from build123d import *

# Parameters (mm, degrees)
BOSS_EXTRUDE1_DEPTH = 10
SKETCH2_R           = 2
CUT_EXTRUDE1_DEPTH  = 30
SKETCH4_W           = 18.757466853
SKETCH4_H           = 10.0829174
CUT_EXTRUDE3_DEPTH  = 5


with BuildPart() as part:
    # Sketch1 → Boss-Extrude1 (new body)
    with BuildSketch(Plane.XY):
        with BuildLine():
            Line((0, -10.891659923), (2, -10.891659923))
            ThreePointArc((2, -10.891659923), (7, -5.891659923), (2, -0.891659923))
            Line((2, -0.891659923), (-20, -0.891659923))
            Line((-20, -0.891659923), (-20, -10.891659923))
            Line((-20, -10.891659923), (0, -10.891659923))
        make_face()
    extrude(amount=BOSS_EXTRUDE1_DEPTH)

    # Sketch2 → Cut-Extrude1 (cut)
    with BuildSketch(Plane.XY.offset(10)):
        with Locations((2, -5.891659923)):
            Circle(SKETCH2_R)
    extrude(amount=-CUT_EXTRUDE1_DEPTH, mode=Mode.SUBTRACT)

    # Sketch4 → Cut-Extrude3 (cut)
    with BuildSketch(Plane.XY.offset(10)):
        with Locations((5.685057141, -5.933118623)):
            Rectangle(SKETCH4_W, SKETCH4_H)
    extrude(amount=-CUT_EXTRUDE3_DEPTH, mode=Mode.SUBTRACT)


solid = part.part
Build history of the part. All positions in model axes, mm. A direction names the side the tool comes from. Round coordinates to 2 decimals unless told otherwise and drop trailing zeros. Write each loop counter-clockwise with the first axis right and the second up, starting at its lowest first coordinate (ties: lowest second). Pieces come first, ordered by that corner, then holes. Notation, with made-up numbers: (-39, 35.25) - (-11, 35.25) arc R16 ccw to (-11, 43.25) - close; hole circle Ø8 at (-40, -3.75). An arc over 180 degrees is marked (long way). One line per question, with ' | ' between items.
1. Tool access for faces 4 (the face through (-12, -6, 10)), 5 (the face through (-1, -6, 5)): list every direction of +Z, -Z, +X, -X, +Y, -Y with a clear straight run to the whole face (end or side of a thin tool).
Results are:
face 4: +Z, +X, -X, +Y, -Y | face 5: +Z, +X, +Y, -Y
2. Band-saw the part on C-C, the plane z = 4. Write the cut outline in (x, y), and give its area (3 significant figures).
Results are:
outline: (-20, -10.89) - (2, -10.89) arc R5 ccw to (2, -0.89) - (-20, -0.89) - close; hole circle Ø4 at (2, -5.89) | area: 247 mm^2
3. Band-saw the part on D-D, the plane z = 7. Write the cut outline in (x, y).
Results are:
outline: (-20, -10.89) - (-3.69, -10.89) - (-3.69, -0.89) - (-20, -0.89) - close
4. Band-saw the part on A-A, the plane x = 0.25. Write the cut outline in (y, z).
Results are:
outline: (-10.89, 0) - (-6.86, 0) - (-6.86, 5) - (-10.89, 5) - close; (-4.92, 0) - (-0.89, 0) - (-0.89, 5) - (-4.92, 5) - close
5. Mould opens along X. For faces 1 (the face through (7, -6, 2)), 2 (the face through (-20, -6, 5)), 3 (the face through (1.74, -3.91, 2.54)) say: released by +X, released by -X, zero draft, split by the parting line, or undercut.
Results are:
face 1: released by +X | face 2: released by -X | face 3: undercut
6. Drill centre lines: line 1 along Y through (x, z) = (2, 1.75); line 2 along X through (y, z) = (-7.25, 5.5); line 3 along Z through (x, y) = (0.5, -10.25). Where is each one in solid material? Low to high. Write a range as from..to.
Results are:
line 1: -10.89..-7.89, -3.89..-0.89 | line 2: -20..-3.69 | line 3: 0..5
7. Band-saw the part on B-B, the plane y = -5.5. Write the cut outline in (x, z), and give its area (3 significant figures).
Results are:
outline: (-20, 0) - (0.04, 0) - (0.04, 5) - (-3.69, 5) - (-3.69, 10) - (-20, 10) - close; (3.96, 0) - (6.98, 0) - (6.98, 5) - (3.96, 5) - close | area: 197 mm^2
8. Drop flat-ended pins along their axis: pin 1 Ø3 at (x, y) = (2, -5.89) entering from -Z; pin 2 Ø1.5 at (y, z) = (-5.5, 7) entering from +X. Give the stop position or say it passes through.
Results are:
pin 1: through | pin 2: x = -3.69
